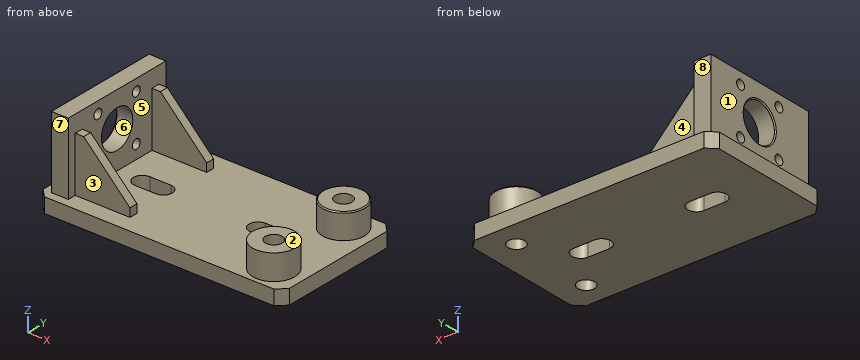
```python
from build123d import *

# Parameters (mm, degrees)
ESQUISSE1_W             = 117
ESQUISSE1_H             = 64
BASE_EXTRUSION_DEPTH    = 7
CHANFREIN1_SIZE         = 4
ESQUISSE2_R             = 10
BOSS_EXTRU_1_DEPTH      = 12
CHANFREIN3_SIZE         = 0.5
ESQUISSE5_R             = 10
BOSS_EXTRU_4_DEPTH      = 12
ESQUISSE7_W             = 8
ESQUISSE7_H             = 56
BOSS_EXTRU_7_DEPTH      = 34
ESQUISSE10_W            = 26
ESQUISSE10_H            = 4
BOSS_EXTRU_9_DEPTH      = 26
CHANFREIN6_SIZE         = 22
ESQUISSE12_W            = 26
ESQUISSE12_H            = 4
BOSS_EXTRU_11_DEPTH     = 26
CHANFREIN7_SIZE         = 22
ESQUISSE13_R            = 9
ENL_V_MAT_EXTRU_1_DEPTH = 118.175082675
CHANFREIN8_SIZE         = 0.5
ESQUISSE3_R             = 4
ENL_V_MAT_EXTRU_2_DEPTH = 98.103038058
ESQUISSE6_R             = 4
ENL_V_MAT_EXTRU_3_DEPTH = 115.893630598
ESQUISSE14_R            = 2.25
ENL_V_MAT_EXTRU_4_DEPTH = 10
ENL_V_MAT_EXTRU_5_DEPTH = 10


with BuildPart() as part:
    # Esquisse1 → Base-Extrusion (new body)
    with BuildSketch(Plane.XY):
        with Locations((-30.5, 0)):
            Rectangle(ESQUISSE1_W, ESQUISSE1_H)
    extrude(amount=BASE_EXTRUSION_DEPTH)

    # Chanfrein1
    chanfrein1_edges = [part.edges().sort_by_distance(p)[0] for p in [
        (-89, 32, 3.5),
        (28, 32, 3.5),
        (28, -32, 3.5),
        (-89, -32, 3.5),
    ]]
    chamfer(chanfrein1_edges, length=CHANFREIN1_SIZE)

    # Esquisse2 → Boss.-Extru.1 (add)
    with BuildSketch(Plane.XY.offset(7)):
        with Locations((14, 20)):
            Circle(ESQUISSE2_R)
    extrude(amount=BOSS_EXTRU_1_DEPTH)

    # Chanfrein3
    chanfrein3_edges = [part.edges().sort_by_distance(p)[0] for p in [
        (4, 20, 19),
    ]]
    chamfer(chanfrein3_edges, length=CHANFREIN3_SIZE)

    # Esquisse5 → Boss.-Extru.4 (add)
    with BuildSketch(Plane(origin=(2.388625814, -32.120396389, 7), x_dir=(1, 0, 0), z_dir=(0, 0, 1))):
        with Locations((11.611374186, 12.120396389)):
            Circle(ESQUISSE5_R)
    extrude(amount=BOSS_EXTRU_4_DEPTH)

    # Esquisse7 → Boss.-Extru.7 (add)
    with BuildSketch(Plane.XY.offset(7)):
        with Locations((-81, 0)):
            Rectangle(ESQUISSE7_W, ESQUISSE7_H)
    extrude(amount=BOSS_EXTRU_7_DEPTH)

    # Esquisse10 → Boss.-Extru.9 (add)
    with BuildSketch(Plane(origin=(-77, 0, 0), x_dir=(0, 0, -1), z_dir=(1, 0, 0))):
        with Locations((-20, -22)):
            Rectangle(ESQUISSE10_W, ESQUISSE10_H)
    extrude(amount=BOSS_EXTRU_9_DEPTH)

    # Chanfrein6
    chanfrein6_edges = [part.edges().sort_by_distance(p)[0] for p in [
        (-51, -22, 33),
    ]]
    chamfer(chanfrein6_edges, length=CHANFREIN6_SIZE)

    # Esquisse12 → Boss.-Extru.11 (add)
    with BuildSketch(Plane(origin=(-77, 31.797692959, 13.355678207), x_dir=(0, 0, -1), z_dir=(1, 0, 0))):
        with Locations((-6.644321793, -9.797692959)):
            Rectangle(ESQUISSE12_W, ESQUISSE12_H)
    extrude(amount=BOSS_EXTRU_11_DEPTH)

    # Chanfrein7
    chanfrein7_edges = [part.edges().sort_by_distance(p)[0] for p in [
        (-51, 22, 33),
    ]]
    chamfer(chanfrein7_edges, length=CHANFREIN7_SIZE)

    # Esquisse13 → Enlèv. mat.-Extru.1 (cut, through all)
    with BuildSketch(Plane(origin=(-77, 0, 0), x_dir=(0, 0, -1), z_dir=(1, 0, 0))):
        with Locations((-24.5, 0)):
            Circle(ESQUISSE13_R)
    extrude(amount=-ENL_V_MAT_EXTRU_1_DEPTH, mode=Mode.SUBTRACT)

    # Chanfrein8
    chanfrein8_edges = [part.edges().sort_by_distance(p)[0] for p in [
        (-85, 0, 33.5),
    ]]
    chamfer(chanfrein8_edges, length=CHANFREIN8_SIZE)

    # Esquisse3 → Enlèv. mat.-Extru.2 (cut, through all)
    with BuildSketch(Plane.XY.offset(19)):
        with Locations((14, 20)):
            Circle(ESQUISSE3_R)
    extrude(amount=-ENL_V_MAT_EXTRU_2_DEPTH, mode=Mode.SUBTRACT)

    # Esquisse6 → Enlèv. mat.-Extru.3 (cut, through all)
    with BuildSketch(Plane(origin=(6.243462417, -28.375733692, 19), x_dir=(1, 0, 0), z_dir=(0, 0, 1))):
        with Locations((7.756537583, 8.375733692)):
            Circle(ESQUISSE6_R)
    extrude(amount=-ENL_V_MAT_EXTRU_3_DEPTH, mode=Mode.SUBTRACT)

    # Esquisse14 → Enlèv. mat.-Extru.4 (cut)
    with BuildSketch(Plane.ZY.offset(85)):
        with Locations((35.5, 11)):
            Circle(ESQUISSE14_R)
        with Locations((13.5, 11)):
            Circle(ESQUISSE14_R)
        with Locations((13.5, -11)):
            Circle(ESQUISSE14_R)
        with Locations((35.5, -11)):
            Circle(ESQUISSE14_R)
    extrude(amount=-ENL_V_MAT_EXTRU_4_DEPTH, mode=Mode.SUBTRACT)

    # Esquisse15 → Enlèv. mat.-Extru.5 (cut)
    with BuildSketch(Plane.XY.offset(7)):
        with BuildLine():
            Line((-10, 4.25), (0, 4.25))
            ThreePointArc((0, 4.25), (4.25, 0), (0, -4.25))
            Line((0, -4.25), (-10, -4.25))
            ThreePointArc((-10, -4.25), (-14.25, 0), (-10, 4.25))
        make_face()
        with BuildLine():
            Line((-65, 4.25), (-55, 4.25))
            ThreePointArc((-55, 4.25), (-50.75, 0), (-55, -4.25))
            Line((-55, -4.25), (-65, -4.25))
            ThreePointArc((-65, -4.25), (-69.25, 0), (-65, 4.25))
        make_face()
    extrude(amount=-ENL_V_MAT_EXTRU_5_DEPTH, mode=Mode.SUBTRACT)


solid = part.part
```
CAD build for the part. Positions are in the model's coordinates, mm. Face numbers are marked on the shaded views. A direction names the side the tool comes from. Round coordinates to 2 decimals unless told otherwise and drop trailing zeros. Order: outer loops, then holes, each group sorted by start corner. A loop starts at its lowest first (then second) coordinate and runs counter-clockwise, first axis right, second up.
Q1. Drop flat-ended pins along their axis: pin 1 (16 mm diameter, centred on x = 10, y = -24, fed in from +Z); pin 2 (14.5 mm diameter, centred on y = 0, z = 24.5, fed in from +X); pin 3 (2.5 mm diameter, centred on y = -11, z = 13.5, fed in from -X); pin 4 (10 mm diameter, centred on x = 4.5, y = -7.5, fed in from +Z). Give the stop position or say it passes through.
Q2. Slice it at D-D (x = -17.5). Write the cut outline in (y, z), and give its area (3 significant figures).
Q3. Two-plate mould, pull along X, no slides. Class the marked faces 1, 2 and 3: pulls with the +X half, pulls with the -X half, needs draft (parallel to the pull), parting line crosses it, or undercut.
Q4. Which spindle directions (+Z, -Z, +X, -X, +Y, -Y) get a long thin tool onto all of the face, cutting with end or side? Do the marked faces 4, 5, 6, 7 and 8. Say none if no direction does.
Q5. Slice it at C-C (z = 35.5). Write the cut outline in (x, y), and give its area (3 significant figures).
Q6. Slice it at A-A (z = 24.5). Write the cut outline in (x, y).
Q7. Wall check: L1, parallel to Y at x = 14, z = 4; L2, parallel to Y at x = 14, z = 12.5; L3, parallel to Y at x = -81.5, z = 35.5. Give the ranges that are in metal, low to high.
Q8. Slice it at B-B (x = -4.5). Write the cut outline in (y, z), and give its area (4 significant figures).
Results below:
1. pin 1: stops at z = 19
1. pin 2: passes through
1. pin 3: stops at x = 7.68
1. pin 4: stops at z = 7
2. outline: (-32, 0) - (32, 0) - (32, 7) - (-32, 7) - close
2. area: 448 mm2
3. face 1: pulls with the -X half
3. face 2: needs draft
3. face 3: undercut
4. face 4: +Z, +Y
4. face 5: +Z
4. face 6: +X, -X
4. face 7: +Z, -X, -Y
4. face 8: +Z, -X, +Y
5. outline: (-85, -28) - (-77, -28) - (-77, -13.25) - (-85, -13.25) - close; (-85, -8.75) - (-77, -8.75) - (-77, 8.75) - (-85, 8.75) - close; (-85, 13.25) - (-77, 13.25) - (-77, 28) - (-85, 28) - close
5. area: 376 mm2
6. outline: (-85, -28) - (-77, -28) - (-77, -24) - (-64.5, -24) - (-64.5, -20) - (-77, -20) - (-77, -9) - (-84.5, -9) - (-85, -9.5) - close; (-85, 9.5) - (-84.5, 9) - (-77, 9) - (-77, 20) - (-64.5, 20) - (-64.5, 24) - (-77, 24) - (-77, 28) - (-85, 28) - close
7. L1: y = -32 to -24, -16 to 16, 24 to 32
7. L2: y = -30 to -24, -16 to -10, 10 to 16, 24 to 30
7. L3: y = -28 to -13.25, -8.75 to 8.75, 13.25 to 28
8. outline: (-32, 0) - (-4.25, 0) - (-4.25, 7) - (-32, 7) - close; (4.25, 0) - (32, 0) - (32, 7) - (4.25, 7) - close
8. area: 388.5 mm2
